Work out the finished part from the listing and answer in its coordinate system (mm). Give positions to 0.01 mm unless a question says otherwise; leave off trailing zeros. Order: outer loops, then holes, each group sorted by start corner. A loop starts at its lowest first (then second) coordinate and runs counter-clockwise, first axis right, second up. Notation, with made-up numbers: (-6, 39) -> (35, 39) arc R21 cw to (35, 78) -> close; hole circle Ø3 at (18.5, 61.25). An arc over 180 degrees is marked (long way). Use a Markdown table: item, result. Add a question column.
```python
from build123d import *

# Parameters (mm, degrees)
F0_W     = 135
F0_H     = 30
F1_DEPTH = 420
F3_DEPTH = 420
F4_W     = 5
F4_H     = 420
F5_DEPTH = 4


with BuildPart() as f1:
    # F0 (on Front) → F1 (new body)
    with BuildSketch(Plane.XZ):
        with Locations((0, 15)):
            Rectangle(F0_W, F0_H)
    extrude(amount=F1_DEPTH)

    # F2 (on face) → F3 (cut)
    with BuildSketch(Plane.XZ.offset(420)):
        Polygon((0, 30), (-52.5, 30), (-52.5, 25), (-55.5, 25), (-55.5, 20), (-52.5, 20), (-52.5, 15), (-55.5, 15), (-55.5, 10), (0, 10), (55.5, 10), (55.5, 15), (52.5, 15), (52.5, 20), (55.5, 20), (55.5, 25), (52.5, 25), (52.5, 30), align=None)
    extrude(amount=-F3_DEPTH, mode=Mode.SUBTRACT)

    # F4 (on face) → F5 (cut)
    with BuildSketch(Plane.XY.offset(30)):
        with Locations((-61.5, -210)):
            Rectangle(F4_W, F4_H)
        with Locations((61.5, -210)):
            Rectangle(F4_W, F4_H)
    extrude(amount=-F5_DEPTH, mode=Mode.SUBTRACT)


solid = f1.part
```
1) Straight lines are drawn through the part: line 1 (X direction, y = -338.5, z = 23); line 2 (X direction, y = -284.5, z = 17); line 3 (Z direction, x = -39.5, y = -232). For each, find the intervals that lie inside material, in ascending order.
2) The part is cut by section B-B, the plane x = -5.5. Determine the outline of the cut face in (y, z).
3) Determine the mould class of faces 1 (the flat face through (-1, 0, 9)), 2 (the flat face through (-1, -213, 10)), 3 (the flat face through (-67.5, -207, 15)) for opening direction X: released by +X, released by -X, zero draft, split by the parting line, or undercut.
4) The part is cut by section A-A, the plane y = -113. Determine the outline of the cut face in (x, z).
5) Flat-ended cylindrical pins translate along their axes: pin 1 (6 mm diameter, centred on x = -10, y = -354.5, fed in from +Z); pin 2 (1.5 mm diameter, centred on x = -61.5, y = -273, fed in from +Z). Find the tip coordinate at first contact, or state that the pin passes through.
A:
| question | item | result |
|---|---|---|
| 1 | line 1 | -67.5 to -55.5, 55.5 to 67.5 |
| 1 | line 2 | -67.5 to -52.5, 52.5 to 67.5 |
| 1 | line 3 | 0 to 10 |
| 2 | outline | (-420, 0) -> (0, 0) -> (0, 10) -> (-420, 10) -> close |
| 3 | face 1 | zero draft |
| 3 | face 2 | undercut |
| 3 | face 3 | released by -X |
| 4 | outline | (-67.5, 0) -> (67.5, 0) -> (67.5, 30) -> (64, 30) -> (64, 26) -> (59, 26) -> (59, 30) -> (52.5, 30) -> (52.5, 25) -> (55.5, 25) -> (55.5, 20) -> (52.5, 20) -> (52.5, 15) -> (55.5, 15) -> (55.5, 10) -> (-55.5, 10) -> (-55.5, 15) -> (-52.5, 15) -> (-52.5, 20) -> (-55.5, 20) -> (-55.5, 25) -> (-52.5, 25) -> (-52.5, 30) -> (-59, 30) -> (-59, 26) -> (-64, 26) -> (-64, 30) -> (-67.5, 30) -> close |
| 5 | pin 1 | z = 10 |
| 5 | pin 2 | z = 26 |
